Can you work these out from the model? Positions are in its coordinate system, mm. A direction names the side the tool comes from. Round coordinates to 2 decimals unless told otherwise and drop trailing zeros. Loops run counter-clockwise (first coordinate to the right, second up) from the corner with the lowest first, then second, coordinate; pieces in that order, holes last.
(1) I want a section at A-A on y = 32.5. Write out the boundary of the cut face in (x, z), plus the area to 3 significant figures.
(2) Will these pins go through, and if not, where does the flat tip stop? pin 1 Ø0.9 at (x, y) = (1, 35) entering from -Z; pin 2 Ø0.9 at (x, y) = (1.5, 42) entering from +Z; pin 3 Ø1.5 at (x, y) = (2, 27.5) entering from -Z; pin 4 Ø2.5 at (y, z) = (2, -26.375) entering from -X.
(3) I want a section at B-B on z = -24. Write out the boundary of the cut face in (x, y), plus the area to 3 significant figures.
(4) Thinking about a two-plate mould opening in Y: for faces 6 (the face through (2, 25.951, 1)), 7 (the face through (0, 19, -9)), 8 (the face through (2, 1, 0)), which applies, released by +Y, released by -Y, zero draft, split by the parting line, or undercut?
(5) I want a section at D-D on y = 2. Write out the boundary of the cut face in (x, z) (3 decimals), plus the area to 3 significant figures.
(6) I want a section at C-C on y = 58.5. Write out the boundary of the cut face in (x, z) (3 decimals).
(7) Which directions (+Z, -Z, +X, -X, +Y, -Y) give clear straight access to the entire face, cutting with the end or side of a thin tool? Please do faces 1 (the face through (2, 17.951, 2)), 2 (the face through (2, -6, -43)), 3 (the face through (2, 17.951, -42)), 4 (the face through (1.48, 63.65, -7.32)), 5 (the face through (2, 46, -36.25)).
(8) If I drill on line 1 along Y through (x, z) = (2.8, -16.5); line 2 along Y through (x, z) = (2, -24); line 3 along Y through (x, z) = (2.65, -16), over which ranges is the centre line in solid material (lowest first)?
Autodesk Inventor part; units mm, degrees
ref_plane "YZ Plane" through (0, 0, 0) normal (1, 0, 0) x (0, 1, 0)
ref_plane "XZ Plane" through (0, 0, 0) normal (0, 1, 0) x (-1, 0, 0)
ref_plane "XY Plane" through (0, 0, 0) normal (0, 0, 1) x (1, 0, 0)
sketch "Boceto1" plane through (0, 0, 0) normal (1, 0, 0) x (0, 1, 0)
  line L0 (0, 0) -> (0, -3)
  line L1 (0, -3) -> (10, -3)
  line L2 (10, -3) -> (10, 0)
  line L3 (10, 0) -> (20, 0)
  line L4 (20, 0) -> (20, -3)
  line L5 (20, -3) -> (30, -3)
  line L6 (30, -33.4269) -> (30, -40)
  line L7 (30, -40) -> (20, -40)
  line L8 (20, -40) -> (20, -43)
  line L9 (20, -43) -> (10, -43)
  line L10 (10, -43) -> (10, -40)
  line L11 (10, -40) -> (0, -40)
  circle A0 centre (15, -21.5) radius 13.175
  arc A1 (0, -9.5731) -> (0, -33.4269) centre (15, -21.5) ccw
  arc A2 (30, -33.4269) -> (30, -9.5731) centre (15, -21.5) ccw
  line L12 (0, -40) -> (0, -33.4269)
  line L13 (0, -9.5731) -> (0, -3)
  line L14 (30, -3) -> (30, -9.5731)
  dimension "d1" = 10
  dimension "d2" = 10
  dimension "d3" = 10
extrude "Extrusión1" add sketch "Boceto1" along normal blind 3
sketch "Boceto2" plane through (3, 0, 0) normal (1, 0, 0) x (0, 0, -1)
  line L0 (3, 10) -> (3, 0)
  line L1 (3, 0) -> (0, 0)
  line L2 (0, 20) -> (0, 10)
  line L3 (0, 0) -> (0, 10)
  line L4 (0, 10) -> (-3, 10)
  line L5 (-3, 10) -> (-3, 20)
  line L6 (-3, 20) -> (0, 20)
  line L7 (0, 20) -> (0, 30)
  line L8 (3, 30) -> (3, 20)
  line L9 (0, 30) -> (3, 30)
  line L10 (3, 30) -> (3, 20)
  line L11 (3, 20) -> (0, 20)
  line L12 (3, 20) -> (0, 20)
  line L13 (0, 20) -> (0, 10)
  line L14 (0, 10) -> (3, 10)
  line L15 (3, 0) -> (3, 10)
  dimension "d11" = 3
extrude "Extrusión2" add sketch "Boceto2" against normal blind 3
sketch "Boceto3" plane through (3, 0, 0) normal (1, 0, 0) x (0, 0, -1)
  line L0 (0, 30) -> (9.5731, 30)
  line L1 (0, 30) -> (9.5731, 30)
  line L2 (40, 30) -> (33.4269, 30)
  line L3 (9.5731, 30) -> (40, 30)
  line L4 (40, 10) -> (40, 0)
  line L5 (40, 30) -> (40, 0)
  line L6 (9.5731, 0) -> (0, 0)
  line L7 (40, 0) -> (0, 0)
  line L8 (0, 30) -> (0, 20)
  line L9 (0, 0) -> (0, 30)
  circle A0 centre (21.5, 15) radius 26.2155
extrude "Extrusión3" cut sketch "Boceto3" against normal blind 10 contours A0 L6 L7 L4 L5 L2 L3 L0 | L8 L9 A0
sketch "Boceto4" plane through (3, 0, 0) normal (1, 0, 0) x (0, 0, -1)
  circle A0 centre (21.5, 15) radius 13.175
  circle A1 centre (21.5, 15) radius 13.175
  circle A2 centre (21.5, 15) radius 3
  point P0 (0, 0)
extrude "Extrusión4" add sketch "Boceto4" against normal blind 3
sketch "Boceto5" plane through (3, 0, 0) normal (1, 0, 0) x (0, 0, -1)
  line L0 (0, 25.951) -> (-3, 25.951)
  line L1 (-3, 25.951) -> (-3, 17.951)
  line L2 (-3, 17.951) -> (0, 17.951)
  line L3 (0, 25.951) -> (0, 17.951)
  line L4 (-3, 11.951) -> (0, 11.951)
  line L5 (0, 11.951) -> (0, 3.951)
  line L6 (0, 3.951) -> (-3, 3.951)
  line L7 (-3, 3.951) -> (-3, 11.951)
  line L8 (40, 0) -> (0, 0)
  line L9 (0, 0) -> (40, 0)
  line L10 (40, 25.951) -> (43, 25.951)
  line L11 (43, 25.951) -> (43, 17.951)
  line L12 (43, 17.951) -> (40, 17.951)
  line L13 (40, 25.951) -> (40, 17.951)
  line L14 (43, 11.951) -> (40, 11.951)
  line L15 (40, 11.951) -> (40, 3.951)
  line L16 (40, 3.951) -> (43, 3.951)
  line L17 (43, 3.951) -> (43, 11.951)
extrude "Extrusión5" add sketch "Boceto5" against normal blind 3
sketch "Boceto6" plane through (3, 0, 0) normal (1, 0, 0) x (0, 0, -1)
  line L0 (31.25, 30) -> (31.25, 55.25)
  line L1 (31.25, 55.25) -> (11.75, 55.25)
  line L2 (11.75, 55.25) -> (11.75, 30)
  line L3 (11.75, 60.25) -> (6.75, 60.25)
  line L4 (31.25, 60.25) -> (36.25, 60.25)
  line L5 (36.25, 60.25) -> (36.25, 30)
  line L6 (31.25, 30) -> (36.25, 30)
  line L7 (31.25, 60.25) -> (11.75, 60.25)
  line L8 (6.75, 60.25) -> (6.75, 30)
  line L9 (6.75, 30) -> (11.75, 30)
  point P0 (0, 0)
  point P1 (21.5, 15)
extrude "Extrusión6" add sketch "Boceto6" against normal blind 3
sketch "Boceto7" plane through (3, 0, 0) normal (1, 0, 0) x (0, 0, -1)
  line L0 (11.75, 30.1448) -> (11.75, 5.25)
  line L1 (11.75, 5.25) -> (31.25, 5.25)
  line L2 (31.25, 5.25) -> (31.25, 30.1448)
  line L3 (31.25, 30.1448) -> (11.75, 30.1448)
  point P0 (0, 0)
  point P1 (21.5, 15)
extrude "Extrusión7" cut sketch "Boceto7" against normal blind 3
sketch "Boceto8" plane through (3, 0, 0) normal (1, 0, 0) x (0, 0, -1)
  line L0 (0, -2.049) -> (-3, -2.049)
  line L1 (-3, -2.049) -> (-3, -10.049)
  line L2 (40, 0) -> (40, -2.049)
  line L3 (40, -2.049) -> (43, -2.049)
  line L4 (43, -2.049) -> (43, -10.049)
  line L5 (43, -10.049) -> (-3, -10.049)
  line L6 (0, 0) -> (0, -2.049)
  line L7 (6.75, 60.25) -> (6.75, 64.25)
  line L8 (36.25, 60.25) -> (36.25, 64.25)
  line L9 (36.25, 64.25) -> (6.75, 64.25)
  line L10 (6.75, 60.25) -> (36.25, 60.25)
  line L11 (6.75, 60.25) -> (36.25, 60.25)
  line L12 (40, 0) -> (0, 0)
  line L13 (0, 0) -> (40, 0)
  point P0 (0, 3.951)
  dimension "d50" = 4
extrude "Extrusión8" add sketch "Boceto8" against normal blind 3
sketch "Boceto9" plane through (3, 0, 0) normal (1, 0, 0) x (0, 0, -1)
  circle A0 centre (26.375, 58.5) radius 1.5
  circle A1 centre (16.625, 58.5) radius 1.5
  circle A2 centre (26.375, 2) radius 1.5
  circle A3 centre (16.625, 2) radius 1.5
  point P0 (0, 0)
extrude "Extrusión9" cut sketch "Boceto9" against normal blind 3
fillet "Empalme1" radius 2 2 edges at (1.5, 64.25, -6.75) (1.5, 64.25, -36.25)
properties part number "cod"
Filled sheet:
1. outline: (0, -36.25) - (3, -36.25) - (3, -31.25) - (0, -31.25) - close; (0, -11.75) - (3, -11.75) - (3, -6.75) - (0, -6.75) - close
1. area: 30.0 mm2
2. pin 1: stops at z = -36.25
2. pin 2: stops at z = -6.75
2. pin 3: stops at z = -40
2. pin 4: passes through
3. outline: (0, -10.05) - (3, -10.05) - (3, 5.25) - (0, 5.25) - close; (0, 55.25) - (3, 55.25) - (3, 64.25) - (0, 64.25) - close
3. area: 72.9 mm2
4. face 6: released by +Y
4. face 7: zero draft
4. face 8: undercut
5. outline: (0, -40) - (3, -40) - (3, -27.875) - (0, -27.875) - close; (0, -24.875) - (3, -24.875) - (3, -18.125) - (0, -18.125) - close; (0, -15.125) - (3, -15.125) - (3, 0) - (0, 0) - close
5. area: 102 mm2
6. outline: (0, -36.25) - (3, -36.25) - (3, -27.875) - (0, -27.875) - close; (0, -24.875) - (3, -24.875) - (3, -18.125) - (0, -18.125) - close; (0, -15.125) - (3, -15.125) - (3, -6.75) - (0, -6.75) - close
7. face 1: +Z, +X, -X
7. face 2: -Z, +X, -X, +Y, -Y
7. face 3: -Z, +X, -X
7. face 4: +Z, +X, -X, +Y
7. face 5: -Z, +X, -X, +Y
8. line 1: y = -10.05 to 0.51, 3.49 to 5.25, 55.25 to 57.01, 59.99 to 64.25
8. line 2: y = -10.05 to 5.25, 55.25 to 64.25
8. line 3: y = -10.05 to 0.64, 3.36 to 5.25, 55.25 to 57.14, 59.86 to 64.25
